Work out the finished part from the listing and answer in its coordinate system (mm). A direction names the side the tool comes from. Give positions to 0.01 mm unless a question says otherwise; leave off trailing zeros. Order: outer loops, then holes, each group sorted by start corner. A loop starts at its lowest first (then second) coordinate and runs counter-clockwise, first axis right, second up. Notation, with made-up numbers: (87, 5) - (100, 5) arc R13 ccw to (100, 30) - close; hole circle Ø11 at (79.25, 0). An arc over 180 degrees is marked (long way). Put each result on its own line as item: value.
```python
from build123d import *

# Parameters (mm, degrees)
SKETCH1_R           = 3.5
EXTRUDE1_DEPTH      = 48
SKETCH3_W           = 8
SKETCH3_H           = 4
EXTRUDE2_DEPTH      = 9
SKETCH4_R           = 2.25
EXTRUDE3_DEPTH      = 2.5
EXTRUDE3_DEPTH_BACK = 6.5
SKETCH5_W           = 8
SKETCH5_H           = 4
EXTRUDE4_DEPTH      = 10
SKETCH6_R           = 2.25
EXTRUDE9_DEPTH      = 2.5000001
EXTRUDE9_DEPTH_BACK = 6.5000001
EXTRUDE10_DEPTH     = 2.25
EXTRUDE11_DEPTH     = 2.25
CHAMFER1_SIZE       = 0.3


with BuildPart() as part:
    # Sketch1 → Extrude1 (new body)
    with BuildSketch(Plane(origin=(0, 0, 0), x_dir=(1, 0, 0), z_dir=(0, 1, 0))):
        with Locations(Location((0, 0, 0), (0, 0, 270))):  # turned: the seam where the file's is
            Circle(SKETCH1_R)
    extrude(amount=EXTRUDE1_DEPTH)

    # Sketch3 → Extrude2 (add)
    with BuildSketch(Plane(origin=(0, 48, 0), x_dir=(1, 0, 0), z_dir=(0, 1, 0))):
        Rectangle(SKETCH3_W, SKETCH3_H)
    extrude(amount=EXTRUDE2_DEPTH)

    # Sketch4 → Extrude3 (cut, two sides)
    with BuildSketch(Plane.XY.offset(2)) as extrude3_sk:
        with Locations((0, 52.25)):
            Circle(SKETCH4_R)
        with BuildLine():
            Line((-7.499970708, 47.987897931), (-8.595568017, 58.173135503))
            Line((-8.595568017, 58.173135503), (8.858273183, 57.495072607))
            Line((8.858273183, 57.495072607), (7.499969018, 47.987553821))
            ThreePointArc((7.499969018, 47.987553821), (4.534958441, 45.531181463), (2.672956888, 48.901345124))
            Line((2.672956888, 48.901345124), (3.097561986, 50.620549251))
            ThreePointArc((3.097561986, 50.620549251), (0, 55.75), (-3.097561986, 50.620549251))
            Line((-3.097561986, 50.620549251), (-2.672956888, 48.901345124))
            ThreePointArc((-2.672956888, 48.901345124), (-4.53465869, 45.531582657), (-7.499970708, 47.987897931))
        make_face()
    extrude(amount=EXTRUDE3_DEPTH, mode=Mode.SUBTRACT)
    extrude(extrude3_sk.sketch, amount=-EXTRUDE3_DEPTH_BACK, mode=Mode.SUBTRACT)

    # Sketch5 → Extrude4 (add)
    with BuildSketch(Plane.XZ):
        Rectangle(SKETCH5_W, SKETCH5_H)
    extrude(amount=EXTRUDE4_DEPTH)

    # Sketch6 → Extrude9 (cut, two sides)
    with BuildSketch(Plane(origin=(0, 0, -2), x_dir=(-1, 0, 0), z_dir=(0, 0, -1))) as extrude9_sk:
        with Locations((0, -4.25)):
            Circle(SKETCH6_R)
        with BuildLine():
            Line((-3.097561986, -2.620549251), (-2.672956888, -0.901345124))
            ThreePointArc((-2.672956888, -0.901345124), (-4.53465869, 2.468417343), (-7.499970708, 0.012102069))
            Line((-7.499970708, 0.012102069), (-8.700661362, -11.644211871))
            Line((-8.700661362, -11.644211871), (9.512578745, -12.130566681))
            Line((9.512578745, -12.130566681), (7.499969018, 0.012446179))
            ThreePointArc((7.499969018, 0.012446179), (4.534958441, 2.468818537), (2.672956888, -0.901345124))
            Line((2.672956888, -0.901345124), (3.097561986, -2.620549251))
            ThreePointArc((3.097561986, -2.620549251), (0, -7.75), (-3.097561986, -2.620549251))
        make_face()
    extrude(amount=EXTRUDE9_DEPTH, mode=Mode.SUBTRACT)
    extrude(extrude9_sk.sketch, amount=-EXTRUDE9_DEPTH_BACK, mode=Mode.SUBTRACT)

    # Sketch7 → Extrude10 (cut)
    with BuildSketch(Plane.XY.offset(3.5)):
        with BuildLine():
            ThreePointArc((0, 46.25), (-1.414213562, 45.664213562), (-2, 44.25))
            Line((-2, 44.25), (-2, 3.75))
            ThreePointArc((-2, 3.75), (-1.414213562, 2.335786438), (0, 1.75))
            ThreePointArc((0, 1.75), (1.414213562, 2.335786438), (2, 3.75))
            Line((2, 3.75), (2, 44.25))
            ThreePointArc((2, 44.25), (1.414213562, 45.664213562), (0, 46.25))
        make_face()
    extrude(amount=-EXTRUDE10_DEPTH, mode=Mode.SUBTRACT)

    # Sketch8 → Extrude11 (cut)
    with BuildSketch(Plane(origin=(0, 0, -3.5), x_dir=(-1, 0, 0), z_dir=(0, 0, -1))):
        with BuildLine():
            Line((-2, 44.25), (-2, 3.75))
            ThreePointArc((-2, 3.75), (0, 1.75), (2, 3.75))
            Line((2, 3.75), (2, 44.25))
            ThreePointArc((2, 44.25), (0, 46.25), (-2, 44.25))
        make_face()
    extrude(amount=-EXTRUDE11_DEPTH, mode=Mode.SUBTRACT)

    # Chamfer1
    chamfer1_edges = [part.edges().sort_by_distance(p)[0] for p in [
        (-2.25, 52.25, -2),
        (-2.25, 52.25, 2),
        (2.25, -4.25, -2),
        (2.25, -4.25, 2),
    ]]
    chamfer(chamfer1_edges, length=CHAMFER1_SIZE)


solid = part.part
```
(1) Given pin 1 (3.5 mm diameter, centred on x = -0.5, y = -3, fed in from +Z); pin 2 (1.3 mm diameter, centred on y = 26.5, z = -2, fed in from +X); pin 3 (4 mm diameter, centred on x = -1.5, z = -1, fed in from +Y); pin 4 (0.8 mm diameter, centred on x = 1, z = -3, fed in from -Y), each flat-ended and moving along its own axis, determine where each tip first touches the part or whether it passes through.
Geometry check:
pin 1: stops at z = 2
pin 2: stops at x = 3.23
pin 3: stops at y = 55.75
pin 4: stops at y = 0
(2) Determine the mould class of faces 6 (the face through (0, 24, -1.25)), 7 (the face through (-2, 50, 2)), 8 (the face through (0, 48, -3)) for opening direction Y: pulls with the +Y half, pulls with the -Y half, needs draft (parallel to the pull), parting line crosses it, or undercut.
Geometry check:
face 6: undercut
face 7: needs draft
face 8: pulls with the +Y half
(3) Section B-B, the plane z = 0 is taken. Write down the section's boundary in (x, y), then the cut area to 3 significant figures.
Geometry check:
outline: (-3.5, 2.01) arc R2.5 cw to (-2.67, -0.9) - (-3.1, -2.62) arc R3.5 ccw (long way) to (3.1, -2.62) - (2.67, -0.9) arc R2.5 cw to (3.5, 2.01) - (3.5, 45.99) arc R2.5 cw to (2.67, 48.9) - (3.1, 50.62) arc R3.5 ccw (long way) to (-3.1, 50.62) - (-2.67, 48.9) arc R2.5 cw to (-3.5, 45.99) - close; hole circle Ø4.5 at (0, -4.25); hole circle Ø4.5 at (0, 52.25)
area: 388 mm²
(4) Straight lines are drawn through the part: line 1 (X direction, y = 31, z = 2.25); line 2 (Y direction, x = 1, z = -1.5); line 3 (Y direction, x = 2, z = 0.25). For each, find the intervals that lie inside material, in ascending order.
Geometry check:
line 1: x = -2.68 to -2, 2 to 2.68
line 2: y = -7.6 to -6.27, -2.23 to 2.02, 45.98 to 50.23, 54.27 to 55.6
line 3: y = -7.12 to -5.28, -3.22 to 51.22, 53.28 to 55.12
(5) Section A-A, the plane y = 52.25 is taken. Write down the section's boundary in (x, z), then the cut area to 3 significant figures.
Geometry check:
outline: (-3.5, -2) - (-2.55, -2) - (-2.25, -1.7) - (-2.25, 1.7) - (-2.55, 2) - (-3.5, 2) - close; (2.25, -1.7) - (2.55, -2) - (3.5, -2) - (3.5, 2) - (2.55, 2) - (2.25, 1.7) - close
area: 9.82 mm²
(6) Section C-C, the plane y = 17 is taken. Write down the section's boundary in (x, z), then the cut area to 3 significant figures.
Geometry check:
outline: (-2, -2.87) - (-2, -1.25) - (2, -1.25) - (2, -2.87) arc R3.5 ccw to (2, 2.87) - (2, 1.25) - (-2, 1.25) - (-2, 2.87) arc R3.5 ccw to start
area: 22.1 mm²
(7) A tool of negligible diameter and unlimited length cuts with its end or side. For faces 1 (the face through (2.365, 23.664, -2.58)), 2 (the face through (0, 0, 3)), 3 (the face through (-2, 24, 2)), 4 (the face through (2.888, -1.773, -0.028)), 5 (the face through (-2.888, 49.773, 0.028)), from which of +Z, -Z, +X, -X, +Y, -Y can it reach the whole face along a straight path? Write none if from no direction.
Geometry check:
face 1: none
face 2: +Z, +X, -X, -Y
face 3: +Z
face 4: +Z, -Z, +X
face 5: +Z, -Z, -X
(8) Section D-D, the plane y = 45 is taken. Write down the section's boundary in (x, z), then the cut area to 3 significant figures.
Geometry check:
outline: (-1.85, -2.97) - (-1.85, -1.25) - (1.85, -1.25) - (1.85, -2.97) arc R3.5 ccw to (1.85, 2.97) - (1.85, 1.25) - (-1.85, 1.25) - (-1.85, 2.97) arc R3.5 ccw to start
area: 23.1 mm²
